```python
from build123d import *

# Parameters (mm, degrees)
SKETCH1_W           = 17.58
SKETCH1_H           = 12.7
SKETCH1_W_2         = 15.98
SKETCH1_H_2         = 30
BOSS_EXTRUDE1_DEPTH = 12.7
SKETCH2_R           = 3.2
CUT_EXTRUDE1_DEPTH  = 174.491786837


with BuildPart() as part:
    # Sketch1 → Boss-Extrude1 (new body)
    with BuildSketch(Plane.XY):
        Polygon((54.94, 144.4), (54.94, 131.7), (72.51, 131.7), (72.51, 78.5), (54.94, 78.5), (54.94, 65.8), (72.51, 65.8), (72.51, 12.7), (54.94, 12.7), (54.94, 0), (39.94, 0), (39.94, 12.7), (22.36, 12.7), (22.36, 0), (-5, 0), (-5, 144.4), (0, 144.4), (0, 157.1), (10, 157.1), (10, 144.4), (22.36, 144.4), (22.36, 131.7), (39.94, 131.7), (39.94, 144.4), align=None)
        with Locations((31.15, 72.15)):
            Rectangle(SKETCH1_W, SKETCH1_H, mode=Mode.SUBTRACT)
        with Locations((7.99, 111.7)):
            Rectangle(SKETCH1_W_2, SKETCH1_H_2, mode=Mode.SUBTRACT)
        with Locations((7.99, 32.7)):
            Rectangle(SKETCH1_W_2, SKETCH1_H_2, mode=Mode.SUBTRACT)
    extrude(amount=BOSS_EXTRUDE1_DEPTH)

    # Sketch2 → Cut-Extrude1 (cut, through all)
    with BuildSketch(Plane.XY.offset(12.7)):
        with Locations((58.14, 131.7)):
            Circle(SKETCH2_R)
        with Locations((58.14, 78.5)):
            Circle(SKETCH2_R)
        with Locations((58.14, 65.8)):
            Circle(SKETCH2_R)
        with Locations((36.74, 78.5)):
            Circle(SKETCH2_R)
        with Locations((36.74, 65.8)):
            Circle(SKETCH2_R)
        with Locations((25.56, 78.5)):
            Circle(SKETCH2_R)
        with Locations((25.56, 65.8)):
            Circle(SKETCH2_R)
        with Locations((25.56, 12.7)):
            Circle(SKETCH2_R)
        with Locations((36.74, 12.7)):
            Circle(SKETCH2_R)
        with Locations((58.14, 12.7)):
            Circle(SKETCH2_R)
        with Locations((36.74, 131.7)):
            Circle(SKETCH2_R)
        with Locations((25.56, 131.7)):
            Circle(SKETCH2_R)
        with Locations((13.2, 144.4)):
            Circle(SKETCH2_R)
        with Locations((15.98, 123.5)):
            Circle(SKETCH2_R)
        with Locations((3.2, 126.7)):
            Circle(SKETCH2_R)
        with Locations((3.2, 96.7)):
            Circle(SKETCH2_R)
        with Locations((15.98, 99.9)):
            Circle(SKETCH2_R)
        with Locations((15.98, 44.5)):
            Circle(SKETCH2_R)
        with Locations((15.98, 20.9)):
            Circle(SKETCH2_R)
        with Locations((3.2, 17.7)):
            Circle(SKETCH2_R)
        with Locations((3.2, 47.7)):
            Circle(SKETCH2_R)
        with Locations((0, 147.6)):
            Circle(SKETCH2_R)
    extrude(amount=-CUT_EXTRUDE1_DEPTH, mode=Mode.SUBTRACT)


solid = part.part
```
Input: part model. Units: mm. Frame: model coordinates. A direction names the side the tool comes from. Round coordinates to 2 decimals unless told otherwise and drop trailing zeros. Loops run counter-clockwise (first coordinate to the right, second up) from the corner with the lowest first, then second, coordinate; pieces in that order, holes last. Notation, with made-up numbers: (-2, 86) -> (16, 86) arc R17 ccw to (16, 117) -> close; hole circle Ø3 at (47, 15). An arc over 180 degrees is marked (long way). Write each question's results on one line, items separated by ' | '.
1. Set-up query: faces 4 (the face through (31, 131.7, 6)), 5 (the face through (47, 144.4, 6)), 6 (the face through (25.6, 81.7, 6.4)). Return all of +Z, -Z, +X, -X, +Y, -Y with unobstructed straight access to the full face (end or side cutting, diameter ignored); none if empty.
Geometry results:
face 4: +Z, -Z, +Y | face 5: +Z, -Z, +X, +Y | face 6: +Z, -Z
2. Section A-A (y = 68.5). Return loops of the section in (x, z), and give its area (3 significant figures).
Geometry results:
outline: (-5, 0) -> (22.36, 0) -> (22.36, 12.7) -> (-5, 12.7) -> close; (39.94, 0) -> (54.94, 0) -> (54.94, 12.7) -> (39.94, 12.7) -> close | area: 538 mm2
3. First-contact query: P1, Ø1.4, axis at x = 31, z = 9.5, coming from the +Y side; P2, Ø4, axis at y = 152.5, z = 9, coming from the +X side; P3, Ø4, axis at x = 32, z = 7.5, coming from the -Y side. Flat tips, straight axial feed; report the tip coordinate or a pass-through.
Geometry results:
P1: y = 131.7 | P2: x = 10 | P3: y = 12.7
4. Section B-B (x = 36.74). Return loops of the section in (y, z), and give its area (3 significant figures).
Geometry results:
outline: (15.9, 0) -> (62.6, 0) -> (62.6, 12.7) -> (15.9, 12.7) -> close; (81.7, 0) -> (128.5, 0) -> (128.5, 12.7) -> (81.7, 12.7) -> close | area: 1,190 mm2
5. Ray query, line 1 (Y direction, x = 8, z = 5); line 2 (X direction, y = 106.5, z = 9.25); line 3 (X direction, y = 77, z = 10.5). Return the intervals inside material, ascending. Write a range as from..to.
Geometry results:
line 1: 0..17.7, 47.7..96.7, 126.7..157.1 | line 2: -5..0, 15.98..72.51 | line 3: -5..22.36, 39.94..54.94
6. Mould query, pull axis Y, two halves, no side actions, for faces 1 (the face through (11, 96.7, 6)), 2 (the face through (36.8, 15.9, 6.4)), 3 (the face through (67, 131.7, 6)). Classes: +Y half, -Y half, draft (parallel to the pull), parting line (faces both ways), or undercut.
Geometry results:
face 1: undercut | face 2: -Y half | face 3: +Y half
7. Section C-C (z = 3.25). State how many separate pieces and enclosed holes the cut face has, and give its area (3 significant figures).
Geometry results:
separate pieces: 1 | enclosed holes: 3 | area: 8,670 mm2
